Autodesk Inventor part; units mm, degrees
ref_plane "YZ Plane" through (0, 0, 0) normal (1, 0, 0) x (0, 1, 0)
ref_plane "XZ Plane" through (0, 0, 0) normal (0, 1, 0) x (-1, 0, 0)
ref_plane "XY Plane" through (0, 0, 0) normal (0, 0, 1) x (1, 0, 0)
sketch "Skizze1" plane through (0, 0, 0) normal (0, 0, 1) x (1, 0, 0)
  circle A0 centre (-15.5, 0) radius 1.5
  circle A1 centre (0, -15.5) radius 1.5
  circle A2 centre (10.9602, 10.9602) radius 1.5
  circle A3 centre (0, 15.5) radius 1.5
  circle A4 centre (15.5, 0) radius 1.5
  circle A5 centre (10.9602, -10.9602) radius 1.5
  circle A6 centre (-10.9602, -10.9602) radius 1.5
  circle A7 centre (-10.9602, 10.9602) radius 1.5
  circle A8 centre (0, 0) radius 11.5
  arc A9 (22.1589, -22.3882) -> (22.1589, 22.3882) centre (0, 0) ccw
  arc A10 (22.1589, 22.3882) -> (22.1589, -22.3882) centre (0, 0) ccw
  circle A11 centre (0, 0) radius 17.5
  point P0 (0, 0)
  dimension "d0" = 35
extrude "Extrusion1" add sketch "Skizze1" along normal blind 9.5 contours A11
sketch "Skizze2" plane through (0, 0, 0) normal (0, 0, -1) x (-1, 0, 0)
  circle A0 centre (0, 0) radius 17.5
  circle A1 centre (0, 0) radius 20
  point P0 (0, 0)
  dimension "d4" = 40
extrude "Extrusion2" add sketch "Skizze2" against normal blind 6
properties part number "RotGear_spacer" material "ABS-Kunststoff"
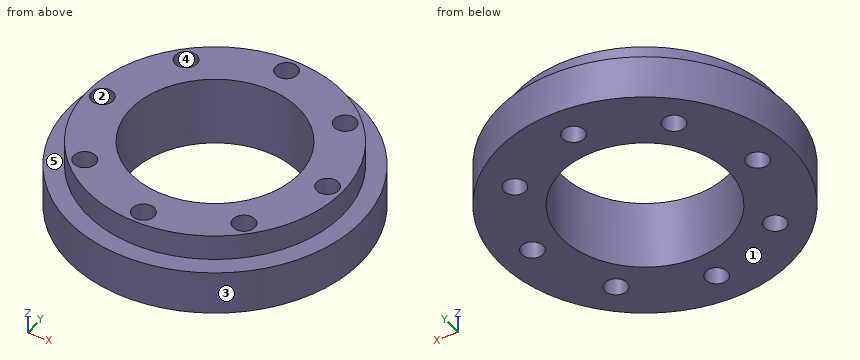
Read the model definition and answer for the solid it produces. Units are mm, in the model's axes. Face numbers are marked on the shaded views. A direction names the side the tool comes from. Give positions to 0.01 mm unless a question says otherwise; leave off trailing zeros. Write each loop counter-clockwise with the first axis right and the second up, starting at its lowest first coordinate (ties: lowest second). Pieces come first, ordered by that corner, then holes. Notation, with made-up numbers: (-25, 37) -> (23, 37) arc R21 cw to (23, 49) -> close; hole circle Ø11 at (66, 66). An arc over 180 degrees is marked (long way). Answer as a JSON object with one key per item and string values.
1) For a pull along X with two mould halves and no side action, classify the marked faces 1, 2 and 3 as pulls with the +X half, pulls with the -X half, needs draft (parallel to the pull), parting line crosses it, or undercut.
Findings below:
{"face 1": "needs draft", "face 2": "undercut", "face 3": "parting line crosses it"}
2) Section C-C on y = 0.5 is taken. Write down the section's boundary in (x, z), then the cut area to 3 significant figures.
Findings below:
{"outline": "(-19.99, 0) -> (-16.91, 0) -> (-16.91, 9.5) -> (-17.49, 9.5) -> (-17.49, 6) -> (-19.99, 6) -> close; (-14.09, 0) -> (-11.49, 0) -> (-11.49, 9.5) -> (-14.09, 9.5) -> close; (11.49, 0) -> (14.09, 0) -> (14.09, 9.5) -> (11.49, 9.5) -> close; (16.91, 0) -> (19.99, 0) -> (19.99, 6) -> (17.49, 6) -> (17.49, 9.5) -> (16.91, 9.5) -> close", "area": "90.3 mm^2"}
3) A tool of negligible diameter and unlimited length cuts with its end or side. For the marked faces 4 and 5, from which of +Z, -Z, +X, -X, +Y, -Y can it reach the whole face along a straight path? Write none if from no direction.
Findings below:
{"face 4": "+Z, -Z", "face 5": "+Z"}
4) Section D-D on z = 7.5 is taken. Count the separate pieces of the cut face and the enclosed holes in it, then the cut area to 3 significant figures.
Findings below:
{"separate pieces": "1", "enclosed holes": "9", "area": "490 mm^2"}
5) Section B-B on y = 15.5 is taken. Write down the section's boundary in (x, z), then the cut area to 3 significant figures.
Findings below:
{"outline": "(-12.64, 0) -> (-1.5, 0) -> (-1.5, 9.5) -> (-8.12, 9.5) -> (-8.12, 6) -> (-12.64, 6) -> close; (1.5, 0) -> (12.64, 0) -> (12.64, 6) -> (8.12, 6) -> (8.12, 9.5) -> (1.5, 9.5) -> close", "area": "180 mm^2"}
6) Section A-A on x = 0 is taken. Write down the section's boundary in (y, z), then the cut area to 3 significant figures.
Findings below:
{"outline": "(-20, 0) -> (-17, 0) -> (-17, 9.5) -> (-17.5, 9.5) -> (-17.5, 6) -> (-20, 6) -> close; (-14, 0) -> (-11.5, 0) -> (-11.5, 9.5) -> (-14, 9.5) -> close; (11.5, 0) -> (14, 0) -> (14, 9.5) -> (11.5, 9.5) -> close; (17, 0) -> (20, 0) -> (20, 6) -> (17.5, 6) -> (17.5, 9.5) -> (17, 9.5) -> close", "area": "87.0 mm^2"}
7) Flat-ended cylindrical pins translate along their axes: pin 1 Ø1 at (x, z) = (-12.5, 4) entering from +Y; pin 2 Ø18.5 at (x, y) = (0, 0) entering from -Z; pin 3 Ø4 at (x, y) = (10.96, -10.96) entering from +Z; pin 4 Ø5 at (x, z) = (-11.5, 7.5) entering from -Y. Find the tip coordinate at first contact, or state that the pin passes through.
Findings below:
{"pin 1": "stops at y = 16", "pin 2": "passes through", "pin 3": "stops at z = 9.5", "pin 4": "stops at y = -17.6"}
8) Straight lines are drawn through the part: probe 1 along X at (y, z) = (12, 1.25); probe 2 along X at (y, z) = (-4, 3.5); probe 3 along Y at (x, z) = (15.5, 4.5). For each, find the intervals that lie inside material, in ascending order. Write a range as from..to.
Findings below:
{"probe 1": "x = -16..-12.04, -9.88..9.88, 12.04..16", "probe 2": "x = -19.6..-10.78, 10.78..19.6", "probe 3": "y = -12.64..-1.5, 1.5..12.64"}
